```python
from build123d import *

# Parameters (mm, degrees)
BOSS_EXTRUDE1_DEPTH   = 17.569451358
BOSS_EXTRUDE1_START   = 17.569451358
BOSS_EXTRUDE1_2_DEPTH = 46.858135107
BOSS_EXTRUDE1_START_2 = -28.07685133
BOSS_EXTRUDE1_3_DEPTH = 23.999999999
CUT_EXTRUDE4_DEPTH    = 110
CUT_EXTRUDE5_DEPTH    = 110
SKETCH7_R             = 2.75
CUT_EXTRUDE6_DEPTH    = 11


with BuildPart() as part:
    # Boss-Extrude1: read off the stored shape, not the designer's step
    # Boss-Extrude1 outline → Boss-Extrude1 (new body)
    with BuildSketch(Plane(origin=(0, 0, 0), x_dir=(1, 0, 0), z_dir=(0, 1, 0))):
        with BuildLine():
            ThreePointArc((-24.671127501, -96.249224292), (-12.589683548, -98.325630278), (-0.686294869, -95.396110217))
            Line((-0.686294869, -95.396110217), (-2.641024782, -40.439954684))
            ThreePointArc((-2.641024782, -40.439954684), (-14.722468735, -38.363548698), (-26.625857414, -41.293068759))
            Line((-26.625857414, -41.293068759), (-24.671127501, -96.249224292))
        make_face()
    extrude(amount=BOSS_EXTRUDE1_DEPTH)

    # Boss-Extrude1 2 outline → Boss-Extrude1 2 (add)
    with BuildSketch(Plane(origin=(0, 0, 0), x_dir=(1, 0, 0), z_dir=(0, 1, 0)).offset(BOSS_EXTRUDE1_START)):
        with BuildLine():
            ThreePointArc((-2.641024782, -40.439954684), (-14.722468735, -38.363548698), (-26.625857414, -41.293068759))
            Line((-26.625857414, -41.293068759), (-24.671127501, -96.249224292))
            ThreePointArc((-24.671127501, -96.249224292), (-12.589683548, -98.325630278), (-0.686294869, -95.396110217))
            Line((-0.686294869, -95.396110217), (-2.641024782, -40.439954684))
        make_face()
    extrude(amount=BOSS_EXTRUDE1_2_DEPTH)

    # Boss-Extrude1 3 outline → Boss-Extrude1 3 (cut)
    with BuildSketch(Plane(origin=(0, 0, 0), x_dir=(0, 1, 0), z_dir=(0.9993680263239928, 0, -0.03554641980970049)).offset(BOSS_EXTRUDE1_START_2)):
        with BuildLine():
            ThreePointArc((17.569338406, 97.816751997), (33.324720821, 67.788721809), (64.427586465, 54.27848788))
            Line((64.427586465, 54.27848788), (64.427586465, 99))
            Line((64.427586465, 99), (17.39740303, 99))
            Line((17.39740303, 99), (17.569338406, 97.816751997))
        make_face()
    extrude(amount=BOSS_EXTRUDE1_3_DEPTH, mode=Mode.SUBTRACT)

    # Sketch5 → Cut-Extrude4 (cut)
    with BuildSketch(Plane(origin=(-28.0591075, 0, 0.998031544), x_dir=(0.035546419809700254, 0, 0.9993680263239927), z_dir=(-0.9993680263239927, 0, 0.035546419809700254))):
        with BuildLine():
            Line((44.891420837, 42.087012188), (56.189188936, 41.889808912))
            ThreePointArc((56.189188936, 41.889808912), (60.605735593, 40.775141371), (64.069709996, 37.817228352))
            Line((64.069709996, 37.817228352), (71.315646663, 80.984453669))
            Line((71.315646663, 80.984453669), (32.067670376, 80.984453669))
            Line((32.067670376, 80.984453669), (32.067670376, 59.188710826))
            ThreePointArc((32.067670376, 59.188710826), (39.974518446, 51.75887054), (44.891420837, 42.087012188))
        make_face()
    extrude(amount=-CUT_EXTRUDE4_DEPTH, mode=Mode.SUBTRACT)

    # Sketch6 → Cut-Extrude5 (cut)
    with BuildSketch(Plane(origin=(-28.0591075, 0, 0.998031544), x_dir=(0.035546419809700254, 0, 0.9993680263239927), z_dir=(-0.9993680263239927, 0, 0.035546419809700254))):
        with BuildLine():
            Line((27.29032593, 61.767303304), (29.792054549, 5.172444286))
            ThreePointArc((29.792054549, 5.172444286), (46.242002949, 34.252323482), (27.29032593, 61.767303304))
        make_face()
    extrude(amount=-CUT_EXTRUDE5_DEPTH, mode=Mode.SUBTRACT)

    # Sketch7 → Cut-Extrude6 (cut)
    with BuildSketch(Plane.XZ):
        with Locations(Location((-14.455870587, 45.858808896, 0), (0, 0, 270))):
            Circle(SKETCH7_R)
        with Locations(Location((-12.856281696, 90.83037008, 0), (0, 0, 270))):
            Circle(SKETCH7_R)
    extrude(amount=-CUT_EXTRUDE6_DEPTH, mode=Mode.SUBTRACT)


solid = part.part
```
Can you work these out from the model? Positions are in its coordinate system, mm. A direction names the side the tool comes from. Round coordinates to 2 decimals unless told otherwise and drop trailing zeros. Order: outer loops, then holes, each group sorted by start corner. A loop starts at its lowest first (then second) coordinate and runs counter-clockwise, first axis right, second up. Notation, with made-up numbers: (71, 9.25) -> (90, 9.25) arc R31 cw to (90, 48.25) -> close; hole circle Ø11 at (19, 66). An arc over 180 degrees is marked (long way). Return JSON: item names as keys, results as strings. Group by question number.
1. We'd pull the mould along Z, two halves only. Please class faces 1 (the face through (-13, 11, 91)), 2 (the face through (-14, 0, 68)), 3 (the face through (-14.55, 5.512, 38.358)): released by +Z, released by -Z, zero draft, split by the parting line, or undercut.
2. If we section it at C-C, the plane z = 52.5: Write out the boundary of the cut face in (x, y).
3. Which directions (+Z, -Z, +X, -X, +Y, -Y) give clear straight access to the entire face, cutting with the end or side of a thin tool? Please do faces 4 (the face through (-12.03, 5.423, 88.207)), 5 (the face through (-14.62, 25.563, 45.964)).
4. I need wall thicknesses on line 1 (Y direction, x = -17, z = 88.5); line 2 (Z direction, x = -11.5, y = 31.5); line 3 (Y direction, x = -14.5, z = 59.5). Which ranges of each line are inside material? Lowest first, please. Write a range as [from, to].
5. If we section it at D-D, the plane y = 39.5: Write out the boundary of the cut face in (x, z), then the cut area to 3 significant figures.
6. If we section it at A-A, the plane y = 3: Write out the boundary of the cut face in (x, z), then the cut area to 3 significant figures.
7. If we section it at B-B, the plane y = 13.5: Write out the boundary of the cut face in (x, z), then the cut area to 3 significant figures.
8. Will these pins go through, and if not, where does the flat tip stop? pin 1 (1.5 mm diameter, centred on x = -3.5, z = 87, fed in from +Y); pin 2 (5 mm diameter, centred on x = -12.86, z = 90.83, fed in from -Y); pin 3 (6 mm diameter, centred on y = 24, z = 69, fed in from +X).
Output values:
{
 "1": {"face 1": "undercut", "face 2": "zero draft", "face 3": "released by -Z"},
 "2": {"outline": "(-26.23, 0) -> (-2.21, 0) -> (-2.21, 41.96) -> (-26.23, 41.97) -> close"},
 "3": {"face 4": "-Y", "face 5": "-Z, -X"},
 "4": {"line 1": "[0, 20.07]", "line 2": "[46.68, 70.02]", "line 3": "[0, 41.45]"},
 "5": {"outline": "(-26.44, 46.53) -> (-2.45, 45.68) -> (-1.85, 62.61) -> (-25.84, 63.46) -> close", "area": "407 mm²"},
 "6": {"outline": "(-26.63, 41.29) arc R30 ccw to (-2.64, 40.44) -> (-0.69, 95.4) arc R30 ccw to (-24.67, 96.25) -> close; hole circle Ø5.5 at (-14.46, 45.86); hole circle Ø5.5 at (-12.86, 90.83)", "area": "1,350 mm²"},
 "7": {"outline": "(-26.63, 41.29) arc R30 ccw to (-24.9, 40.53) -> (-4.42, 39.8) arc R30 ccw to (-2.64, 40.44) -> (-0.69, 95.4) arc R30 ccw to (-24.67, 96.25) -> close", "area": "1,380 mm²"},
 "8": {"pin 1": "y = 20.74", "pin 2": "y = 11", "pin 3": "x = -1.52"}
}
